Build history of the part. All positions in model axes, mm. Give positions to 0.01 mm unless a question says otherwise; leave off trailing zeros. Loops run counter-clockwise (first coordinate to the right, second up) from the corner with the lowest first, then second, coordinate; pieces in that order, holes last. Notation, with made-up numbers: (58.25, 50) -> (91.25, 50) arc R25 ccw to (91.25, 76) -> close; hole circle Ø1 at (-28, 67). An arc over 180 degrees is marked (long way). Answer in a Markdown table with one row per item. Add a question column.
from build123d import *

# Parameters (mm, degrees)
SKETCH1_W           = 132
SKETCH1_H           = 60
BOSS_EXTRUDE1_DEPTH = 1
SKETCH4_W           = 11.62
SKETCH4_H           = 9
SKETCH4_W_2         = 14.16
SKETCH4_W_3         = 34.5
CUT_EXTRUDE3_DEPTH  = 2
SKETCH11_W          = 1
SKETCH11_H          = 20
CUT_EXTRUDE6_DEPTH  = 2


with BuildPart() as part:
    # Sketch1 → Boss-Extrude1 (new body)
    with BuildSketch(Plane.XY):
        with Locations((17.755849622, 9.633412311)):
            Rectangle(SKETCH1_W, SKETCH1_H)
    extrude(amount=BOSS_EXTRUDE1_DEPTH)

    # Sketch4 → Cut-Extrude3 (cut, through all)
    with BuildSketch(Plane(origin=(0, 0, 0), x_dir=(-1, 0, 0), z_dir=(0, 0, -1))):
        with Locations((-41.525849622, -8.521305626)):
            Rectangle(SKETCH4_W, SKETCH4_H)
        with Locations((-20.885849622, -8.521305626)):
            Rectangle(SKETCH4_W_2, SKETCH4_H)
        with Locations((5.444150378, -8.521305626)):
            Rectangle(SKETCH4_W_3, SKETCH4_H)
    extrude(amount=-CUT_EXTRUDE3_DEPTH, mode=Mode.SUBTRACT)

    # Sketch11 → Cut-Extrude6 (cut, through all)
    with BuildSketch(Plane(origin=(0, 0, 0), x_dir=(-1, 0, 0), z_dir=(0, 0, -1))):
        with Locations((-53.992691727, 19.633412311)):
            Rectangle(SKETCH11_W, SKETCH11_H)
        with Locations((-58.255849622, 19.633412311)):
            Rectangle(SKETCH11_W, SKETCH11_H)
        with Locations((-49.729533832, 19.633412311)):
            Rectangle(SKETCH11_W, SKETCH11_H)
        with Locations((-45.466375937, 19.633412311)):
            Rectangle(SKETCH11_W, SKETCH11_H)
        with Locations((-41.203218043, 19.633412311)):
            Rectangle(SKETCH11_W, SKETCH11_H)
        with Locations((-36.940060148, 19.633412311)):
            Rectangle(SKETCH11_W, SKETCH11_H)
        with Locations((-32.676902253, 19.633412311)):
            Rectangle(SKETCH11_W, SKETCH11_H)
        with Locations((-28.413744358, 19.633412311)):
            Rectangle(SKETCH11_W, SKETCH11_H)
        with Locations((-24.150586464, 19.633412311)):
            Rectangle(SKETCH11_W, SKETCH11_H)
        with Locations((-19.887428569, 19.633412311)):
            Rectangle(SKETCH11_W, SKETCH11_H)
        with Locations((-15.624270674, 19.633412311)):
            Rectangle(SKETCH11_W, SKETCH11_H)
        with Locations((-11.36111278, 19.633412311)):
            Rectangle(SKETCH11_W, SKETCH11_H)
        with Locations((-7.097954885, 19.633412311)):
            Rectangle(SKETCH11_W, SKETCH11_H)
        with Locations((-2.83479699, 19.633412311)):
            Rectangle(SKETCH11_W, SKETCH11_H)
        with Locations((1.428360905, 19.633412311)):
            Rectangle(SKETCH11_W, SKETCH11_H)
        with Locations((5.691518799, 19.633412311)):
            Rectangle(SKETCH11_W, SKETCH11_H)
        with Locations((9.954676694, 19.633412311)):
            Rectangle(SKETCH11_W, SKETCH11_H)
        with Locations((14.217834589, 19.633412311)):
            Rectangle(SKETCH11_W, SKETCH11_H)
        with Locations((18.480992484, 19.633412311)):
            Rectangle(SKETCH11_W, SKETCH11_H)
        with Locations((22.744150378, 19.633412311)):
            Rectangle(SKETCH11_W, SKETCH11_H)
    extrude(amount=-CUT_EXTRUDE6_DEPTH, mode=Mode.SUBTRACT)


solid = part.part
(1) Saw through at A-A, the plane y = -7. List the corners of the cut face in (x, z).
(2) Saw through at B-B, the plane z = 0.35. State how many separate pieces and enclosed holes the cut face has, then the cut area to 3 significant figures.
(3) Wall check: line 1 along Y through (x, z) = (-9.5, 0.2); line 2 along Y through (x, z) = (20.5, 0.85); line 3 along X through (y, z) = (-6, 0.8). Give the ranges that are in metal, low to high. Write a range as from..to.
Worked answers:
| question | item | result |
|---|---|---|
| 1 | outline | (-48.24, 0) -> (-22.69, 0) -> (-22.69, 1) -> (-48.24, 1) -> close; (11.81, 0) -> (13.81, 0) -> (13.81, 1) -> (11.81, 1) -> close; (27.97, 0) -> (35.72, 0) -> (35.72, 1) -> (27.97, 1) -> close; (47.34, 0) -> (83.76, 0) -> (83.76, 1) -> (47.34, 1) -> close |
| 2 | separate pieces | 1 |
| 2 | enclosed holes | 23 |
| 2 | area | 6,980 mm^2 |
| 3 | line 1 | -20.37..-13.02, -4.02..9.63, 29.63..39.63 |
| 3 | line 2 | -20.37..-13.02, -4.02..39.63 |
| 3 | line 3 | -48.24..-22.69, 11.81..13.81, 27.97..35.72, 47.34..83.76 |
